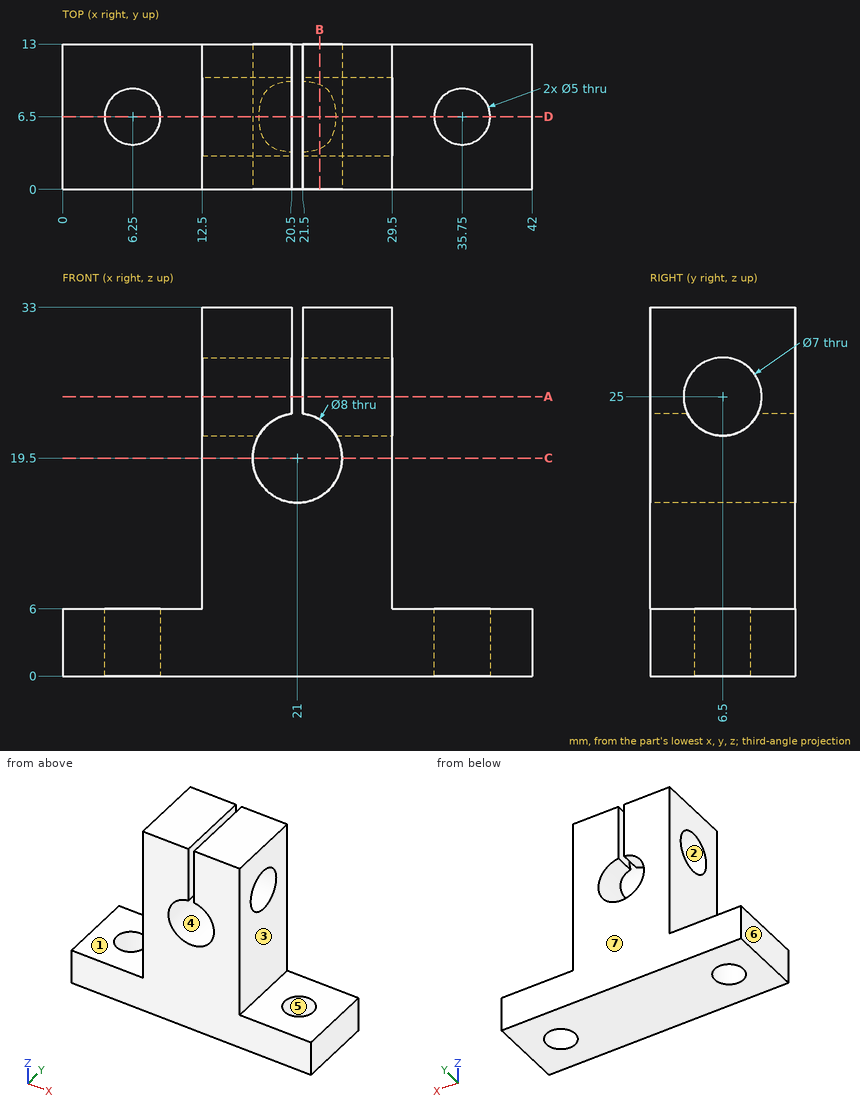
Here's the drawing with two shaded views (mm, measured from the low corner). I have some questions. A direction names the side the tool comes from. Give positions to 0.01 mm unless a question says otherwise; leave off trailing zeros. Loops run counter-clockwise (first coordinate to the right, second up) from the corner with the lowest first, then second, coordinate; pieces in that order, holes last. Notation, with made-up numbers: M 20.25,-30.75 L 35.25,-30.75 A17 ccw 35.25,-5.75 Z; hole C 45.25,19 d4. An arc over 180 degrees is marked long. One line per item, written item: value.
(1) Suppose I cut it at D-D on y = 6.5. List the corners of the cut face in (x, z) for me, plus the area to 3 significant figures.
Returned:
outline: M 0,0 L 3.75,0 L 3.75,6 L 0,6 Z; M 8.75,0 L 33.25,0 L 33.25,6 L 29.5,6 L 29.5,21.5 L 24.46,21.5 A4 cw long 17.54,21.5 L 12.5,21.5 L 12.5,6 L 8.75,6 Z; M 12.5,28.5 L 20.5,28.5 L 20.5,33 L 12.5,33 Z; M 21.5,28.5 L 29.5,28.5 L 29.5,33 L 21.5,33 Z; M 38.25,0 L 42,0 L 42,6 L 38.25,6 Z
area: 487 mm^2
(2) Will these pins go through, and if not, where does the flat tip stop? pin 1 (4 mm diameter, centred on y = 4.5, z = 21.5, fed in from +X); pin 2 (6 mm diameter, centred on x = 28, y = 6.5, fed in from -Z); pin 3 (2 mm diameter, centred on y = 6.5, z = 8.5, fed in from -X); pin 4 (4 mm diameter, centred on x = 6.25, y = 6.5, fed in from +Z).
Returned:
pin 1: x = 29.5
pin 2: z = 0
pin 3: x = 12.5
pin 4: through
(3) We'd pull the mould along X, two halves only. Please class the marked faces 4, 5, 6 and 7: released by +X, released by -X, zero draft, split by the parting line, or undercut.
Returned:
face 4: undercut
face 5: undercut
face 6: released by -X
face 7: zero draft
(4) Suppose I cut it at B-B on x = 23. List the corners of the cut face in (y, z) for me, plus the area to 3 significant figures.
Returned:
outline: M 0,0 L 13,0 L 13,16.04 L 0,16.04 Z; M 0,22.96 L 3.65,22.96 A3.5 cw long 9.35,22.96 L 13,22.96 L 13,33 L 0,33 Z
area: 306 mm^2
(5) I need wall thicknesses on line 1 (X direction, y = 12, z = 31); line 2 (Y direction, x = 24.25, z = 25); line 3 (Y direction, x = 35.75, z = 1.6). Which ranges of each line are inside material? Lowest first, please.
Returned:
line 1: 12.5 to 20.5, 21.5 to 29.5
line 2: 0 to 3, 10 to 13
line 3: 0 to 4, 9 to 13
(6) Suppose I cut it at C-C on z = 19.5. List the corners of the cut face in (x, y) for me.
Returned:
outline: M 12.5,0 L 17,0 L 17,13 L 12.5,13 Z; M 25,0 L 29.5,0 L 29.5,13 L 25,13 Z
(7) Which directions (+Z, -Z, +X, -X, +Y, -Y) give clear straight access to the entire face, cutting with the end or side of a thin tool? Please do the marked faces 1, 2 and 3.
Returned:
face 1: +Z, -X, +Y, -Y
face 2: +X, -X
face 3: +Z, +X, +Y, -Y
(8) Suppose I cut it at A-A on z = 25. List the corners of the cut face in (x, y) for me, plus the area to 3 significant figures.
Returned:
outline: M 12.5,0 L 20.5,0 L 20.5,3 L 12.5,3 Z; M 12.5,10 L 20.5,10 L 20.5,13 L 12.5,13 Z; M 21.5,0 L 29.5,0 L 29.5,3 L 21.5,3 Z; M 21.5,10 L 29.5,10 L 29.5,13 L 21.5,13 Z
area: 96.0 mm^2
